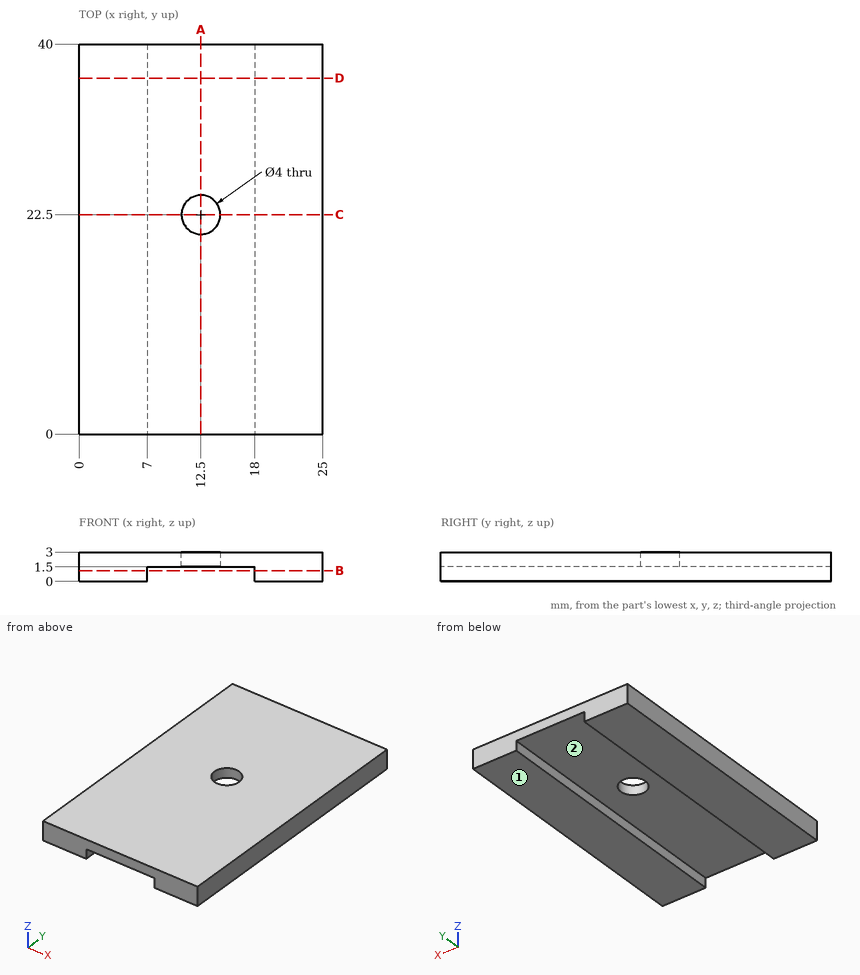
Check sheet for the drawn part. Datum: minimum x, y, z corner. Units: mm. A direction names the side the tool comes from. Round coordinates to 2 decimals unless told otherwise and drop trailing zeros. Write each loop counter-clockwise with the first axis right and the second up, starting at its lowest first coordinate (ties: lowest second). Pieces come first, ordered by that corner, then holes. Notation, with made-up numbers: (73.25, 51.25) -> (103.25, 51.25) arc R31 ccw to (103.25, 77.25) -> close; hole circle Ø1 at (40, 46). An arc over 180 degrees is marked (long way). One line per item, written item: value. Start each with the question number.
(1) Cross-section at D-D, the plane y = 36.5. Record the cut outline in (x, z).
(2) Scan lines: line 1 (Y direction, x = 12.5, z = 1.7); line 2 (Z direction, x = 9.25, y = 36.5); line 3 (X direction, y = 25, z = 0.45). Record each from-to range of solid material in increasing order. Write a range as [from, to].
(3) Cross-section at C-C, the plane y = 22.5. Record the cut outline in (x, z).
(4) Access from +Z, -Z, +X, -X, +Y, -Y to the whole of each face (thin tool, end or side, straight path). Record for the marked faces 1 and 2.
(5) Cross-section at A-A, the plane x = 12.5. Record the cut outline in (y, z), and give its area (3 significant figures).
(6) Cross-section at B-B, the plane z = 1.1. Record the cut outline in (x, y), and give its area (3 significant figures).
(7) Go/stop test with flat-tipped pins: pin 1 Ø1.5 at (x, z) = (21, 2) entering from -Y; pin 2 Ø5.5 at (x, y) = (12.5, 19) entering from -Z. Record where each tip stops, or that it passes through.
Answer:
1. outline: (0, 0) -> (7, 0) -> (7, 1.5) -> (18, 1.5) -> (18, 0) -> (25, 0) -> (25, 3) -> (0, 3) -> close
2. line 1: [0, 20.5], [24.5, 40]
2. line 2: [1.5, 3]
2. line 3: [0, 7], [18, 25]
3. outline: (0, 0) -> (7, 0) -> (7, 1.5) -> (10.5, 1.5) -> (10.5, 3) -> (0, 3) -> close; (14.5, 1.5) -> (18, 1.5) -> (18, 0) -> (25, 0) -> (25, 3) -> (14.5, 3) -> close
4. face 1: -Z, +X, -X, +Y, -Y
4. face 2: -Z, +Y, -Y
5. outline: (0, 1.5) -> (20.5, 1.5) -> (20.5, 3) -> (0, 3) -> close; (24.5, 1.5) -> (40, 1.5) -> (40, 3) -> (24.5, 3) -> close
5. area: 54.0 mm²
6. outline: (0, 0) -> (7, 0) -> (7, 40) -> (0, 40) -> close; (18, 0) -> (25, 0) -> (25, 40) -> (18, 40) -> close
6. area: 560 mm²
7. pin 1: y = 0
7. pin 2: z = 1.5
